Design review of the part built by this model. Coordinates are the model's own, in mm. A direction names the side the tool comes from. Round coordinates to 2 decimals unless told otherwise and drop trailing zeros. Loops run counter-clockwise (first coordinate to the right, second up) from the corner with the lowest first, then second, coordinate; pieces in that order, holes last. Notation, with made-up numbers: (42, 36) -> (50, 36) arc R13 cw to (50, 40) -> close; hole circle Ø1 at (-36.75, 30.5). An arc over 180 degrees is marked (long way). Use a Markdown table: item, result. Add a question column.
from build123d import *

# Parameters (mm, degrees)
BOSS_EXTRUDE1_DEPTH      = 10
BOSS_EXTRUDE1_DEPTH_BACK = 50
FILLET1_R                = 2
BOSS_EXTRUDE2_START      = -5
SKETCH3_R                = 2.4
BOSS_EXTRUDE2_DEPTH      = 5
FILLET2_R                = 22


with BuildPart() as part:
    # Sketch2 → Boss-Extrude1 (new, two sides: drawn at the far end of the back side and taken through both)
    with BuildSketch(Plane(origin=(0, 0, 0), x_dir=(1, 0, 0), z_dir=(0, 1, 0)).offset(-BOSS_EXTRUDE1_DEPTH_BACK)):
        with BuildLine():
            ThreePointArc((-22.5, 98.49115601), (0, 101.0285), (22.5, 98.49115601))
            ThreePointArc((22.5, 98.49115601), (0, 107.821909931), (-22.5, 98.49115601))
        make_face()
    extrude(amount=BOSS_EXTRUDE1_DEPTH + BOSS_EXTRUDE1_DEPTH_BACK)

    # Fillet1
    fillet1_edges = [part.edges().sort_by_distance(p)[0] for p in [
        (22.5, -20, -98.49115601),
        (-22.5, -20, -98.49115601),
    ]]
    fillet(fillet1_edges, radius=FILLET1_R)

    # Sketch3 → Boss-Extrude2 (add)
    with BuildSketch(Plane(origin=(0, 0, 0), x_dir=(1, 0, 0), z_dir=(0, 1, 0)).offset(BOSS_EXTRUDE2_START)):
        with BuildLine():
            ThreePointArc((14.341382747, 100.005412619), (0, 101.0285), (-14.341382747, 100.005412619))
            ThreePointArc((-14.341382747, 100.005412619), (0, 89.401404079), (14.341382747, 100.005412619))
        make_face()
        with Locations(Location((0, 94.415, 0), (0, 0, 270))):
            Circle(SKETCH3_R, mode=Mode.SUBTRACT)
    extrude(amount=BOSS_EXTRUDE2_DEPTH)

    # Fillet2
    # the kernel refuses this fillet: 22 mm, written as the material it adds along each edge
    with BuildSketch(Plane(origin=(0, -5, 0), x_dir=(0.6340991791841111, 0, -0.7732517254801548), z_dir=(0.7732517254801548, 0, 0.6340991791841111))) as fillet2_piece_1_section:
        with BuildLine():
            CenterArc((101.0285 - FILLET2_R, -FILLET2_R), FILLET2_R, 0, 90)
            Line((101.0285 - FILLET2_R, 0), (101.0285, 0))
            Line((101.0285, 0), (101.0285, -FILLET2_R))
        make_face()
    fillet2_piece_1 = revolve(axis=Axis((0, -5, 0), (0, 1, 0)), revolution_arc=78.706408495, mode=Mode.PRIVATE)
    fillet2_piece_1 = fillet2_piece_1 & Plane(origin=(0, -11.179397571, -104.401404079), x_dir=(-0.9560921831070281, 0, 0.29306609732556405), z_dir=(0, -1, 0)) * Cylinder(15, 405, mode=Mode.PRIVATE)
    fillet2_piece_1 = fillet2_piece_1 - Plane(origin=(0, -11.179397571, -94.415), x_dir=(0, 0, 1), z_dir=(0, -1, 0)) * Cylinder(2.4, 405, mode=Mode.PRIVATE)
    add(fillet2_piece_1)


solid = part.part
1. To check wall thickness, follow probe 1 along Z at (x, y) = (1, -14); probe 2 along Z at (x, y) = (5, -44); probe 3 along X at (y, z) = (-10, -102.5). State the ranges of each line that lie inside material, in increasing order. Write a range as from..to.
2. Consider section A-A on x = 0. State the section outline as (y, z) points (1 decimal), plus the area to 3 significant figures.
3. For faces 1 (the face through (0, -50, -104)), 2 (the face through (-0.2, -38.66, -101.03)), list the 3-axis set-ups (+Z, -Z, +X, -X, +Y, -Y) from which the entire face can be reached by the end or side of a thin tool; tool diameter is ignored.
4. Mouldability with a two-part tool opening along X and no side actions: class faces 3 (the face through (0, 10, -104)), 4 (the face through (-0.2, 4.93, -101.03)), 5 (the face through (0.23, -20.42, -107.82)) as +X half, -X half, draft (parallel to the pull), parting line (faces both ways), or undercut.
5. Insertion check: P1, Ø6, axis at x = -1.5, y = -4, coming from the -Z side; P2, Ø3, axis at x = -10.5, y = -18.5, coming from the -Z side; P3, Ø2, axis at x = -8.5, y = -28, coming from the -Z side; P4, Ø1, axis at x = 12.5, z = -94.5, coming from the +Y side. Each pin has a flat end and moves straight along its axis. Give the tip position at first contact, or say it passes through.
Verdict:
| question | item | result |
|---|---|---|
| 1 | probe 1 | z = -107.81..-96.77 |
| 1 | probe 2 | z = -107.43..-100.9 |
| 1 | probe 3 | x = -16.56..16.56 |
| 2 | outline | (-50, -107.8) -> (10, -107.8) -> (10, -101) -> (0, -101) -> (0, -96.8) -> (-14.1, -96.8) arc R22 cw to (-27, -101) -> (-50, -101) -> close; (-9.2, -92) -> (0, -92) -> (0, -89.4) -> (-7.6, -89.4) arc R22 cw to start |
| 2 | area | 506 mm² |
| 3 | face 1 | +Z, -Z, +X, -X, -Y |
| 3 | face 2 | +Z, -Y |
| 4 | face 3 | draft |
| 4 | face 4 | undercut |
| 4 | face 5 | parting line |
| 5 | P1 | stops at z = -107.82 |
| 5 | P2 | stops at z = -106.52 |
| 5 | P3 | stops at z = -106.92 |
| 5 | P4 | passes through |
